from build123d import *

# Parameters (mm, degrees)
SKETCH1_W           = 101.6
SKETCH1_H           = 63.5
BOSS_EXTRUDE1_DEPTH = 3.175
SKETCH2_W           = 101.6
SKETCH2_H           = 63.5
SKETCH2_W_2         = 95.25
SKETCH2_H_2         = 57.15
BOSS_EXTRUDE3_DEPTH = 25.4
SKETCH3_R           = 2.141141326
CUT_EXTRUDE1_DEPTH  = 3.175
SKETCH5_R           = 4.675
SKETCH5_R_2         = 3.175
BOSS_EXTRUDE4_DEPTH = 25.4


with BuildPart() as part:
    # Sketch1 → Boss-Extrude1 (new body)
    with BuildSketch(Plane(origin=(0, 0, 0), x_dir=(1, 0, 0), z_dir=(0, 1, 0))):
        with Locations((11.723076923, 23.795054945)):
            Rectangle(SKETCH1_W, SKETCH1_H)
    extrude(amount=BOSS_EXTRUDE1_DEPTH)

    # Sketch2 → Boss-Extrude3 (add)
    with BuildSketch(Plane(origin=(0, 3.175, 0), x_dir=(1, 0, 0), z_dir=(0, 1, 0))):
        with Locations((11.723076923, 23.795054945)):
            Rectangle(SKETCH2_W, SKETCH2_H)
        with Locations((11.723076923, 23.795054945)):
            Rectangle(SKETCH2_W_2, SKETCH2_H_2, mode=Mode.SUBTRACT)
    extrude(amount=BOSS_EXTRUDE3_DEPTH)

    # Sketch3 → Cut-Extrude1 (cut)
    with BuildSketch(Plane.XZ):
        with Locations((47.814406836, -23.777289581)):
            Circle(SKETCH3_R)
    extrude(amount=-CUT_EXTRUDE1_DEPTH, mode=Mode.SUBTRACT)

    # Sketch5 → Boss-Extrude4 (add)
    with BuildSketch(Plane(origin=(0, 3.175, 0), x_dir=(1, 0, 0), z_dir=(0, 1, 0))):
        with Locations((-30.726923077, 47.190054945)):
            Circle(SKETCH5_R)
        with Locations((-30.726923077, 47.190054945)):
            Circle(SKETCH5_R_2, mode=Mode.SUBTRACT)
        with Locations((54.168076923, 0.400054945)):
            Circle(SKETCH5_R)
        with Locations((54.168076923, 0.400054945)):
            Circle(SKETCH5_R_2, mode=Mode.SUBTRACT)
    extrude(amount=BOSS_EXTRUDE4_DEPTH)


solid = part.part
Can you work these out from the model? Positions are in its coordinate system, mm. A direction names the side the tool comes from. Coordinates: 2 decimals unless noted, no trailing zeros. Write each loop counter-clockwise with the first axis right and the second up, starting at its lowest first coordinate (ties: lowest second). Pieces come first, ordered by that corner, then holes. Notation, with made-up numbers: (67, 50) -> (112, 50) arc R17 ccw to (112, 57) -> close; hole circle Ø9 at (4, 16.5). An arc over 180 degrees is marked (long way). Answer as CSV lines item,"result".
1) If we section it at C-C on x = 4.5: Please give me the cut outline in (y, z) (3 decimals).
Check result:
outline,"(0, -55.545) -> (28.575, -55.545) -> (28.575, -52.37) -> (3.175, -52.37) -> (3.175, 4.78) -> (28.575, 4.78) -> (28.575, 7.955) -> (0, 7.955) -> close"
2) If we section it at A-A on z = -15.5: Please give me the cut outline in (x, y) (3 decimals).
Check result:
outline,"(-39.077, 0) -> (62.523, 0) -> (62.523, 28.575) -> (59.348, 28.575) -> (59.348, 3.175) -> (-35.902, 3.175) -> (-35.902, 28.575) -> (-39.077, 28.575) -> close"
3) If I drill on line 1 (X direction, y = 18.5, z = -47); line 2 (X direction, y = 12, z = -33.5); line 3 (Z direction, x = 24.5, y = 26.75), over which ranges is the centre line in solid material (lowest first)? Write a range as from..to.
Check result:
line 1,"-39.08..-35.9, -35.4..-33.9, -27.56..-26.06, 59.35..62.52"
line 2,"-39.08..-35.9, 59.35..62.52"
line 3,"-55.55..-52.37, 4.78..7.95"
4) If we mould it in two halves opening along X, with no side actions, what happens to faces 1 (the flat face through (-32, 28.575, -44)), 2 (the flat face through (59.348, 16, -23)), 3 (the flat face through (-39.077, 14, -23))? For each: +X half, -X half, draft (parallel to the pull), parting line (faces both ways), or undercut.
Check result:
face 1,"draft"
face 2,"undercut"
face 3,"-X half"
5) Will these pins go through, and if not, where does the flat tip stop? P1, Ø5.5, axis at x = 54.17, z = -0.4, coming from the +Y side (3 decimals); P2, Ø3.5, axis at x = 47.81, z = -23.78, coming from the +Y side.
Check result:
P1,"y = 3.175"
P2,"through"
6) If we section it at B-B on y = 7: Please give me the cut outline in (x, z) (3 decimals).
Check result:
outline,"(-39.077, -55.545) -> (62.523, -55.545) -> (62.523, 7.955) -> (-39.077, 7.955) -> close; circle Ø9.35 at (-30.727, -47.19); circle Ø9.35 at (54.168, -0.4); hole (-35.902, -52.37) -> (59.348, -52.37) -> (59.348, 4.78) -> (-35.902, 4.78) -> close; hole circle Ø6.35 at (-30.727, -47.19); hole circle Ø6.35 at (54.168, -0.4)"
7) On a 3-axis mill with a long thin cutter (end or side, diameter ignored), from which of +Z, -Z, +X, -X, +Y, -Y can I reach the whole of each face in a straight line? I mean faces 4 (the flat face through (11, 16, 4.78)), 5 (the cylindrical face through (47.35, 1.565, -25.868)). Say none if no direction works.
Check result:
face 4,"+Y"
face 5,"+Y, -Y"
